Work out the finished part from the listing and answer in its coordinate system (mm). A direction names the side the tool comes from. Round coordinates to 2 decimals unless told otherwise and drop trailing zeros. Order: outer loops, then holes, each group sorted by start corner. A loop starts at its lowest first (then second) coordinate and runs counter-clockwise, first axis right, second up. Notation, with made-up numbers: (-18.5, 24) -> (-8.5, 24) arc R22 ccw to (-8.5, 48) -> close; hole circle Ø7 at (31.25, -31). An arc over 180 degrees is marked (long way). Use one line per item in the form item = value.
```python
from build123d import *

# Parameters (mm, degrees)
SKETCH1_W                    = 50
SKETCH1_H                    = 40
BASE_FLANGE1_DEPTH           = 1.5
EDGE_FLANGE1_STRIP_CUT_DEPTH = 40
EDGE_FLANGE1_DEPTH           = 40
EDGE_FLANGE2_START           = -25.866025404
EDGE_FLANGE2_DEPTH           = 2.598076212
EDGE_FLANGE2_START_2         = -23.267949192
EDGE_FLANGE2_2_DEPTH         = 48.267949192
EDGE_FLANGE2_3_DEPTH         = 50.866025404
EDGE_FLANGE2_START_3         = -21
EDGE_FLANGE2_4_DEPTH         = 4
SKETCH12_R                   = 1.5
CUT_EXTRUDE1_DEPTH           = 10
FILLET1_R                    = 10
FILLET2_R                    = 5


with BuildPart() as part:
    # Base-Flange1: sheet metal written as solids
    # Sketch1 → Base-Flange1 (new body)
    with BuildSketch(Plane.XY):
        Rectangle(SKETCH1_W, SKETCH1_H)
    extrude(amount=BASE_FLANGE1_DEPTH)

    # Edge-Flange1: sheet metal written as solids
    # Edge-Flange1 strip (on a plane across the edge) → Edge-Flange1 strip cut (cut)
    with BuildSketch(Plane(origin=(-25, 20, 1.5), x_dir=(0.8660254037844364, 0, 0.5000000000000041), z_dir=(0, -1, 0))):
        Polygon((-9.642304845, 3.834936491), (0.75, -2.165063509), (1.5, -0.866025404), (-8.892304845, 5.133974596), align=None)
    extrude(amount=EDGE_FLANGE1_STRIP_CUT_DEPTH, mode=Mode.SUBTRACT)

    # Edge-Flange1 section (on a plane across the edge) → Edge-Flange1 (add)
    with BuildSketch(Plane(origin=(-25, 20, 1.5), x_dir=(0.8660254037844364, 0, 0.5000000000000041), z_dir=(0, -1, 0))):
        with BuildLine():
            Line((-1.5, 1.732050808), (-1.5, 48.633974596))
            Line((-1.5, 48.633974596), (0, 48.633974596))
            Line((0, 48.633974596), (0, 1.732050808))
            ThreePointArc((0, 1.732050808), (0.401923789, 0.232050808), (1.5, -0.866025404))
            Line((1.5, -0.866025404), (0.75, -2.165063509))
            ThreePointArc((0.75, -2.165063509), (-0.897114317, -0.517949192), (-1.5, 1.732050808))
        make_face()
    extrude(amount=EDGE_FLANGE1_DEPTH)

    # Edge-Flange2: read off the stored shape, not the designer's step
    # Edge-Flange2 outline → Edge-Flange2 (cut)
    with BuildSketch(Plane.YZ.offset(EDGE_FLANGE2_START)):
        with BuildLine():
            Line((-17, 0), (-17, 1.5))
            ThreePointArc((-17, 1.5), (-19.121320344, 2.378679656), (-20, 4.5))
            Line((-20, 4.5), (-20, 16.5))
            Line((-20, 16.5), (-21.5, 16.5))
            Line((-21.5, 16.5), (-21.5, 4.5))
            ThreePointArc((-21.5, 4.5), (-21.107919181, 2.662882693), (-20, 1.145898034))
            ThreePointArc((-20, 1.145898034), (-18.605699404, 0.296224385), (-17, 0))
        make_face()
    extrude(amount=EDGE_FLANGE2_DEPTH, mode=Mode.SUBTRACT)

    # Edge-Flange2 2 outline → Edge-Flange2 2 (add)
    with BuildSketch(Plane.YZ.offset(EDGE_FLANGE2_START_2)):
        with BuildLine():
            Line((-17, 0), (-17, 1.5))
            ThreePointArc((-17, 1.5), (-19.121320344, 2.378679656), (-20, 4.5))
            Line((-20, 4.5), (-20, 16.5))
            Line((-20, 16.5), (-21.5, 16.5))
            Line((-21.5, 16.5), (-21.5, 4.5))
            ThreePointArc((-21.5, 4.5), (-21.107919181, 2.662882693), (-20, 1.145898034))
            ThreePointArc((-20, 1.145898034), (-18.605699404, 0.296224385), (-17, 0))
        make_face()
    extrude(amount=EDGE_FLANGE2_2_DEPTH)

    # Edge-Flange2 3 outline → Edge-Flange2 3 (cut)
    with BuildSketch(Plane.YZ.offset(EDGE_FLANGE2_START)):
        with BuildLine():
            ThreePointArc((-17, 0), (-18.605699404, 0.296224385), (-20, 1.145898034))
            Line((-20, 1.145898034), (-20, 0))
            Line((-20, 0), (-17, 0))
        make_face()
    extrude(amount=EDGE_FLANGE2_3_DEPTH, mode=Mode.SUBTRACT)

    # Edge-Flange2 4 outline → Edge-Flange2 4 (cut)
    with BuildSketch(Plane(origin=(0, 0, 0), x_dir=(1, 0, 0), z_dir=(0, 1, 0)).offset(EDGE_FLANGE2_START_3)):
        with BuildLine():
            ThreePointArc((-25.866025404, -3), (-24.767949192, -1.901923789), (-23.267949192, -1.5))
            Line((-23.267949192, -1.5), (-23.267949192, 0))
            ThreePointArc((-23.267949192, 0), (-25.517949192, -0.602885683), (-27.165063509, -2.25))
            Line((-27.165063509, -2.25), (-25.866025404, -3))
        make_face()
    extrude(amount=EDGE_FLANGE2_4_DEPTH, mode=Mode.SUBTRACT)

    # Sketch12 → Cut-Extrude1 (cut)
    with BuildSketch(Plane(origin=(0, -20, 0), x_dir=(1, 0, 0), z_dir=(0, 1, 0))):
        with Locations(Location((-17.5, -11.5, 0), (0, 0, 270))):
            Circle(SKETCH12_R)
        with Locations(Location((17.5, -11.5, 0), (0, 0, 270))):
            Circle(SKETCH12_R)
    extrude(amount=-CUT_EXTRUDE1_DEPTH, mode=Mode.SUBTRACT)

    # Fillet1
    fillet1_edges = [part.edges().sort_by_distance(p)[0] for p in [
        (-49.966506351, 20, 43.243257487),
        (-49.966506351, -20, 43.243257487),
        (25, 20, 0.75),
    ]]
    fillet(fillet1_edges, radius=FILLET1_R)

    # Fillet2
    # the kernel refuses this fillet: 5 mm, written as the material it takes off along each edge
    with BuildSketch(Plane(origin=(-37.086630924, -20, -3.478219621), x_dir=(-0.5000000001953341, 0, 0.8660254036716625), z_dir=(0.8660254036716625, 0, 0.5000000001953341))) as fillet2_piece_1:
        with BuildLine():
            CenterArc((4.582575695, -5), FILLET2_R, 90, 66.421821522)
            Line((0, -3), (0, 0))
            Line((0, 0), (4.582575695, 0))
        make_face()
    extrude(amount=24.412878474, mode=Mode.SUBTRACT)
    with BuildSketch(Plane(origin=(-23.267949192, -7.5, 16.5), x_dir=(1, 0, 0), z_dir=(0, -1, 0)), Plane(origin=(25, -7.5, 16.5), x_dir=(0, 0, -1), z_dir=(0, -1, 0))) as fillet2_piece_2:
        with BuildLine():
            CenterArc((FILLET2_R, -FILLET2_R), FILLET2_R, 90, 90)
            Line((0, -FILLET2_R), (0, 0))
            Line((0, 0), (FILLET2_R, 0))
        make_face()
    extrude(amount=26.5, mode=Mode.SUBTRACT)


solid = part.part
```
Item 1: The part is cut by section D-D, the plane y = -15. Give the vertices of the cut face in (x, z), and give its area (3 significant figures).
Findings:
outline = (-49.95, 41.71) -> (-27.17, 2.25) arc R4.5 ccw to (-23.27, 0) -> (25, 0) -> (25, 1.5) -> (-23.27, 1.5) arc R3 cw to (-25.87, 3) -> (-48.65, 42.46) -> close
area = 147 mm^2
Item 2: Flat-ended cylindrical pins translate along their axes: P1, Ø6, axis at y = -10, z = 27, coming from the -X side; P2, Ø5, axis at x = -36.5, z = 24.5, coming from the -Y side; P3, Ø10, axis at y = -5, z = 19.5, coming from the +X side. Find the tip coordinate at first contact, or state that the pin passes through.
Findings:
P1 = -43.19
P2 = -20
P3 = -32.51
Item 3: For faces 4 (the flat face through (-23.268, -20.3, 5.8)), 5 (the cylindrical face through (-25.489, 1.759, 0.586)), determine the directions among +Z, -Z, +X, -X, +Y, -Y from which every point of the face is accessible in a straight line to the end or side of a thin tool.
Findings:
face_4 = +Z, -Z, -X, -Y
face_5 = -Z, -X, +Y, -Y
Item 4: The part is cut by section A-A, the plane y = -2.5. Give the vertices of the cut face in (x, z).
Findings:
outline = (-50.62, 42.87) -> (-27.17, 2.25) arc R4.5 ccw to (-23.27, 0) -> (25, 0) -> (25, 1.5) -> (-23.27, 1.5) arc R3 cw to (-25.87, 3) -> (-49.32, 43.62) -> close
Item 5: The part is cut by section B-B, the plane x = 17.5. Give the vertices of the cut face in (y, z), and give its area (3 significant figures).
Findings:
outline = (-21.5, 4.5) arc R4.5 ccw to (-17, 0) -> (19.68, 0) -> (19.68, 1.5) -> (-17, 1.5) arc R3 cw to (-20, 4.5) -> (-20, 10) -> (-21.5, 10) -> close; (-21.5, 13) -> (-20, 13) -> (-20, 16.5) -> (-21.5, 16.5) -> close
area = 77.4 mm^2
Item 6: Consider line 1 along X through (y, z) = (-20.8, 11.5); line 2 along Z through (x, y) = (-20.5, 14.5); line 3 along Y through (x, z) = (9.5, 11.5). Determine where each line is inside the solid, lowest interval first.
Findings:
line_1 = -23.27 to -19, -16 to 16, 19 to 25
line_2 = 0 to 1.5
line_3 = -21.5 to -20
Item 7: The part is cut by section C-C, the plane x = -10. Give the vertices of the cut face in (y, z).
Findings:
outline = (-21.5, 4.5) arc R4.5 ccw to (-17, 0) -> (20, 0) -> (20, 1.5) -> (-17, 1.5) arc R3 cw to (-20, 4.5) -> (-20, 16.5) -> (-21.5, 16.5) -> close
Item 8: Determine the mould class of faces 1 (the flat face through (1, -21, 16.5)), 2 (the cylindrical face through (22.15, 16.99, 0.76)), 3 (the cylindrical face through (18.51, -20.74, 10.39)) for opening direction Z: released by +Z, released by -Z, zero draft, split by the parting line, or undercut.
Findings:
face_1 = released by +Z
face_2 = zero draft
face_3 = undercut
